Check sheet for the modelled part. Datum: model origin and axes. Units: mm. A direction names the side the tool comes from. Give positions to 0.01 mm unless a question says otherwise; leave off trailing zeros. Write each loop counter-clockwise with the first axis right and the second up, starting at its lowest first coordinate (ties: lowest second). Pieces come first, ordered by that corner, then holes. Notation, with made-up numbers: (-4, -24) -> (9, -24) arc R26 ccw to (9, -3) -> close; hole circle Ø10 at (13.25, -28.5). An arc over 180 degrees is marked (long way). Write each question's results on one line, items separated by ' | '. Start each with the question number.
```python
from build123d import *

# Parameters (mm, degrees)
SKETCH1_R           = 1.625
SKETCH1_R_2         = 3.5
SKETCH1_R_3         = 1.125
SKETCH1_W           = 8
SKETCH1_H           = 4
BOSS_EXTRUDE1_DEPTH = 2
BOSS_EXTRUDE2_DEPTH = 1.5
SKETCH4_R           = 1
CUT_EXTRUDE1_DEPTH  = 52.758903682


with BuildPart() as part:
    # Sketch1 → Boss-Extrude1 (new body)
    with BuildSketch(Plane.XY):
        with BuildLine():
            Line((-4.833560916, 12.25), (5.166439084, 12.25))
            Line((5.166439084, 12.25), (40.166439084, 12.25))
            Line((40.166439084, 12.25), (40.166439084, 9.964216866))
            ThreePointArc((40.166439084, 9.964216866), (50.16018383, -0.389429797), (39.459588189, -10.010769942))
            Line((39.459588189, -10.010769942), (39.459588189, -12.25))
            Line((39.459588189, -12.25), (5.166439084, -12.25))
            Line((5.166439084, -12.25), (-4.833560916, -12.25))
            Line((-4.833560916, -12.25), (-24.833560916, -12.25))
            Line((-24.833560916, -12.25), (-24.833560916, -8.25))
            Line((-24.833560916, -8.25), (4.166439084, -8.25))
            Line((4.166439084, -8.25), (4.166439084, 8.25))
            Line((4.166439084, 8.25), (-24.833560916, 8.25))
            Line((-24.833560916, 8.25), (-24.833560916, 12.25))
            Line((-24.833560916, 12.25), (-4.833560916, 12.25))
        make_face()
        with Locations((40.166439084, 6.964216866)):
            Circle(SKETCH1_R, mode=Mode.SUBTRACT)
        with Locations((47.166439084, -0.035783134)):
            Circle(SKETCH1_R, mode=Mode.SUBTRACT)
        with Locations((40.166439084, -7.035783134)):
            Circle(SKETCH1_R, mode=Mode.SUBTRACT)
        with Locations((33.166439084, -0.035783134)):
            Circle(SKETCH1_R, mode=Mode.SUBTRACT)
        with Locations((40.166439084, -0.035783134)):
            Circle(SKETCH1_R_2, mode=Mode.SUBTRACT)
        with Locations((-2.833560916, 9.964216866)):
            Circle(SKETCH1_R_3, mode=Mode.SUBTRACT)
        with Locations((-2.833560916, -10.035783134)):
            Circle(SKETCH1_R_3, mode=Mode.SUBTRACT)
        with Locations((-22.833560916, 9.964216866)):
            Circle(SKETCH1_R_3, mode=Mode.SUBTRACT)
        with Locations((-22.833560916, -10.035783134)):
            Circle(SKETCH1_R_3, mode=Mode.SUBTRACT)
        with Locations((20.166471095, 7)):
            Rectangle(SKETCH1_W, SKETCH1_H, mode=Mode.SUBTRACT)
        with Locations((20.166471095, -7)):
            Rectangle(SKETCH1_W, SKETCH1_H, mode=Mode.SUBTRACT)
    extrude(amount=BOSS_EXTRUDE1_DEPTH)

    # Sketch2 → Boss-Extrude2 (add)
    with BuildSketch(Plane.XY.offset(2)):
        Polygon((-24.833560916, 12.25), (7.666439084, 12.25), (7.313013637, -12.25), (-24.833560916, -12.25), (-24.833560916, -8.25), (4.166439084, -8.25), (4.166439084, 8.25), (-24.833560916, 8.25), align=None)
    extrude(amount=BOSS_EXTRUDE2_DEPTH)

    # Sketch4 → Cut-Extrude1 (cut, through all)
    with BuildSketch(Plane(origin=(0, 0, 0), x_dir=(-1, 0, 0), z_dir=(0, 0, -1))):
        with Locations((2.833560916, 9.964216866)):
            Circle(SKETCH4_R)
        with Locations((2.833560916, -10.035783134)):
            Circle(SKETCH4_R)
        with Locations((22.833560916, -10.035783134)):
            Circle(SKETCH4_R)
        with Locations((22.833560916, 9.964216866)):
            Circle(SKETCH4_R)
    extrude(amount=-CUT_EXTRUDE1_DEPTH, mode=Mode.SUBTRACT)


solid = part.part
```
Item 1: Set-up check for faces 4 (the cylindrical face through (-22.31, 8.97, 0.99)), 5 (the flat face through (20, 9, 1)), 6 (the flat face through (1, -12.25, 1)): record each of +Z, -Z, +X, -X, +Y, -Y from which the full face is reachable in a straight line by a thin tool's end or side.
Item 2: Section check B-B on x = 18.5. Record the boundary of the cut face in (y, z), then the cut area to 3 significant figures.
Item 3: Depth check by flat-ended pin: pin 1 Ø6 at (x, y) = (18, 6.5) entering from +Z; pin 2 Ø1.9 at (x, y) = (40.17, -7.04) entering from -Z. Enter the tip coordinate at first touch or a pass-through.
Item 4: Thickness scan on probe 1 along Y at (x, z) = (0, 0.8); probe 2 along Y at (x, z) = (-3, 1.05); probe 3 along X at (y, z) = (10.5, 2.05). Record the ranges inside material, lowest first. Write a range as from..to.
Item 5: Section check A-A on x = 3. Record the boundary of the cut face in (y, z), then the cut area to 3 significant figures.
Item 6: Section check C-C on z = 2.85. Record the boundary of the cut face in (x, y), then the cut area to 3 significant figures.
Item 7: Mould release check, pull along X, two halves, no side actions. Record for faces 1 (the flat face through (-10, 8.25, 2)), 2 (the flat face through (4.166, 0, 2)), 3 (the flat face through (24.166, -7, 1)): pulls with the +X half, pulls with the -X half, needs draft (parallel to the pull), parting line crosses it, or undercut.
Item 8: Section check D-D on y = -4.25. Record the boundary of the cut face in (x, z).
Check sheet entries:
1) face 4: -Z | face 5: +Z, -Z | face 6: +Z, -Z, +X, -X, -Y
2) outline: (-12.25, 0) -> (-9, 0) -> (-9, 2) -> (-12.25, 2) -> close; (-5, 0) -> (5, 0) -> (5, 2) -> (-5, 2) -> close; (9, 0) -> (12.25, 0) -> (12.25, 2) -> (9, 2) -> close | area: 33.0 mm^2
3) pin 1: stops at z = 2 | pin 2: passes through
4) probe 1: y = -12.25..-8.25, 8.25..12.25 | probe 2: y = -12.25..-11.15, -8.92..-8.25, 8.25..8.85, 11.08..12.25 | probe 3: x = -24.83..-23.68, -21.99..-3.68, -1.99..7.64
5) outline: (-12.25, 0) -> (-8.25, 0) -> (-8.25, 3.5) -> (-12.25, 3.5) -> close; (8.25, 0) -> (12.25, 0) -> (12.25, 3.5) -> (8.25, 3.5) -> close | area: 28.0 mm^2
6) outline: (-24.83, -12.25) -> (7.31, -12.25) -> (7.67, 12.25) -> (-24.83, 12.25) -> (-24.83, 8.25) -> (4.17, 8.25) -> (4.17, -8.25) -> (-24.83, -8.25) -> close; hole circle Ø2 at (-22.83, -10.04); hole circle Ø2 at (-22.83, 9.96); hole circle Ø2 at (-2.83, -10.04); hole circle Ø2 at (-2.83, 9.96) | area: 301 mm^2
7) face 1: needs draft | face 2: pulls with the -X half | face 3: undercut
8) outline: (4.17, 0) -> (49.24, 0) -> (49.24, 2) -> (7.43, 2) -> (7.43, 3.5) -> (4.17, 3.5) -> close
